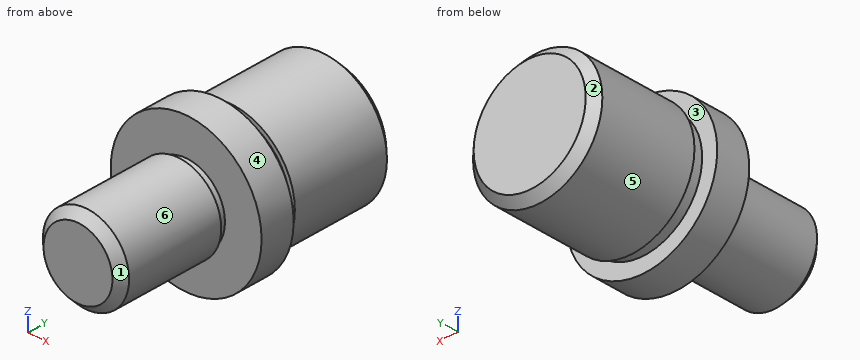
from build123d import *

# Parameters (mm, degrees)
SKETCH_1_R          = 17.5
EXTRUDE_1_DEPTH     = 63
SKETCH_2_OUTSIDE_W  = 53.024
SKETCH_2_OUTSIDE_H  = 53.024
SKETCH_2_OUTSIDE_R  = 15
CUT_EXTRUDE_1_DEPTH = 25
SKETCH_3_OUTSIDE_W  = 53.024
SKETCH_3_OUTSIDE_H  = 53.024
SKETCH_3_OUTSIDE_R  = 14
CUT_EXTRUDE_2_DEPTH = 3
SKETCH_4_OUTSIDE_W  = 53.024
SKETCH_4_OUTSIDE_H  = 53.024
SKETCH_4_OUTSIDE_R  = 10
CUT_EXTRUDE_3_DEPTH = 25
SKETCH_5_OUTSIDE_W  = 53.024
SKETCH_5_OUTSIDE_H  = 53.024
SKETCH_5_OUTSIDE_R  = 9
CUT_EXTRUDE_4_DEPTH = 2
CHAMFER_1_SIZE      = 2


with BuildPart() as part:
    # 草图1 → 凸台-拉伸1 (new body)
    with BuildSketch(Plane(origin=(0, 0, 0), x_dir=(1, 0, 0), z_dir=(0, 1, 0))):
        Circle(SKETCH_1_R)
    extrude(amount=EXTRUDE_1_DEPTH)

    # 草图2 outside → 切除-拉伸1 (cut)
    with BuildSketch(Plane(origin=(0, 63, 0), x_dir=(1, 0, 0), z_dir=(0, 1, 0))):
        Rectangle(SKETCH_2_OUTSIDE_W, SKETCH_2_OUTSIDE_H)
        Circle(SKETCH_2_OUTSIDE_R, mode=Mode.SUBTRACT)
    extrude(amount=-CUT_EXTRUDE_1_DEPTH, mode=Mode.SUBTRACT)

    # 草图3 outside → 切除-拉伸2 (cut)
    with BuildSketch(Plane(origin=(0, 38, 0), x_dir=(1, 0, 0), z_dir=(0, 1, 0))):
        Rectangle(SKETCH_3_OUTSIDE_W, SKETCH_3_OUTSIDE_H)
        Circle(SKETCH_3_OUTSIDE_R, mode=Mode.SUBTRACT)
    extrude(amount=-CUT_EXTRUDE_2_DEPTH, mode=Mode.SUBTRACT)

    # 草图4 outside → 切除-拉伸3 (cut)
    with BuildSketch(Plane.XZ):
        Rectangle(SKETCH_4_OUTSIDE_W, SKETCH_4_OUTSIDE_H)
        Circle(SKETCH_4_OUTSIDE_R, mode=Mode.SUBTRACT)
    extrude(amount=-CUT_EXTRUDE_3_DEPTH, mode=Mode.SUBTRACT)

    # 草图5 outside → 切除-拉伸4 (cut)
    with BuildSketch(Plane.XZ.offset(-25)):
        Rectangle(SKETCH_5_OUTSIDE_W, SKETCH_5_OUTSIDE_H)
        Circle(SKETCH_5_OUTSIDE_R, mode=Mode.SUBTRACT)
    extrude(amount=-CUT_EXTRUDE_4_DEPTH, mode=Mode.SUBTRACT)

    # 倒角1
    chamfer_1_edges = [part.edges().sort_by_distance(p)[0] for p in [
        (-15, 63, 0),
        (-10, 0, 0),
    ]]
    chamfer(chamfer_1_edges, length=CHAMFER_1_SIZE)


solid = part.part
Work out the finished part from the listing and answer in its coordinate system (mm). Face numbers are marked on the shaded views. A direction names the side the tool comes from. Give positions to 0.01 mm unless a question says otherwise; leave off trailing zeros. Order: outer loops, then holes, each group sorted by start corner. A loop starts at its lowest first (then second) coordinate and runs counter-clockwise, first axis right, second up. Notation, with made-up numbers: (-39, 10.5) -> (12, 10.5) arc R10 cw to (12, 14.5) -> close; hole circle Ø4 at (-3.75, -31). An arc over 180 degrees is marked (long way). Answer as a JSON object with one key per item and string values. Group by question number.
1. Section A-A on z = 0 is taken. Determine the outline of the cut face in (x, y).
2. Section B-B on x = 0 is taken. Determine the outline of the cut face in (y, z).
3. The mould has two halves that part along Y. Classify the marked faces 1, 2 and 3: released by +Y, released by -Y, zero draft, split by the parting line, or undercut.
4. Flat-ended cylindrical pins translate along their axes: pin 1 Ø12 at (x, y) = (13, 41.5) entering from -Z; pin 2 Ø1.5 at (y, z) = (52.5, 4.5) entering from +X; pin 3 Ø1 at (x, y) = (7, 44) entering from -Z. Find the tip coordinate at first contact, or state that the pin passes through.
5. Section D-D on y = 52 is taken. Determine the outline of the cut face in (x, z).
6. A tool of negligible diameter and unlimited length cuts with its end or side. For the marked faces 4, 5 and 6, from which of +Z, -Z, +X, -X, +Y, -Y can it reach the whole face along a straight path? Write none if from no direction.
7. Consider line 1 along Y through (x, z) = (-12, -12); line 2 along Z through (x, y) = (0, 18.5); line 3 along Z through (x, y) = (-12, 60). Determine where each line is inside the solid, lowest interval first. Write a range as [from, to].
8. Section C-C on y = 36 is taken. Determine the outline of the cut face in (x, z).
Result sheet:
{
 "1": {"outline": "(-17.5, 27) -> (-9, 27) -> (-9, 25) -> (-10, 25) -> (-10, 2) -> (-8, 0) -> (8, 0) -> (10, 2) -> (10, 25) -> (9, 25) -> (9, 27) -> (17.5, 27) -> (17.5, 35) -> (14, 35) -> (14, 38) -> (15, 38) -> (15, 61) -> (13, 63) -> (-13, 63) -> (-15, 61) -> (-15, 38) -> (-14, 38) -> (-14, 35) -> (-17.5, 35) -> close"},
 "2": {"outline": "(0, -8) -> (2, -10) -> (25, -10) -> (25, -9) -> (27, -9) -> (27, -17.5) -> (35, -17.5) -> (35, -14) -> (38, -14) -> (38, -15) -> (61, -15) -> (63, -13) -> (63, 13) -> (61, 15) -> (38, 15) -> (38, 14) -> (35, 14) -> (35, 17.5) -> (27, 17.5) -> (27, 9) -> (25, 9) -> (25, 10) -> (2, 10) -> (0, 8) -> close"},
 "3": {"face 1": "released by -Y", "face 2": "released by +Y", "face 3": "undercut"},
 "4": {"pin 1": "stops at z = -13.27", "pin 2": "stops at x = 14.52", "pin 3": "stops at z = -13.52"},
 "5": {"outline": "circle Ø30 at (0, 0)"},
 "6": {"face 4": "+Y, -Y", "face 5": "+Y", "face 6": "-Y"},
 "7": {"line 1": "y = [27, 35]", "line 2": "z = [-10, 10]", "line 3": "z = [-9, 9]"},
 "8": {"outline": "circle Ø28 at (0, 0)"}
}
